from build123d import *

# Parameters (mm, degrees)
F0_R     = 20
F0_R_2   = 2
F0_R_3   = 12.5
F1_DEPTH = 2


with BuildPart() as f1:
    # F0 (on Top) → F1 (new body)
    with BuildSketch(Plane.XY):
        Circle(F0_R)
        with Locations((-11.490485, -11.490485)):
            Circle(F0_R_2, mode=Mode.SUBTRACT)
        with Locations((-6.218606, -15.013042)):
            Circle(F0_R_2, mode=Mode.SUBTRACT)
        with Locations((-15.013042, -6.218606)):
            Circle(F0_R_2, mode=Mode.SUBTRACT)
        with Locations((0, -16.25)):
            Circle(F0_R_2, mode=Mode.SUBTRACT)
        with Locations((6.218606, -15.013042)):
            Circle(F0_R_2, mode=Mode.SUBTRACT)
        with Locations((11.490485, -11.490485)):
            Circle(F0_R_2, mode=Mode.SUBTRACT)
        with Locations((15.013042, -6.218606)):
            Circle(F0_R_2, mode=Mode.SUBTRACT)
        with Locations((-16.25, 0)):
            Circle(F0_R_2, mode=Mode.SUBTRACT)
        with Locations((-15.013042, 6.218606)):
            Circle(F0_R_2, mode=Mode.SUBTRACT)
        with Locations((-11.490485, 11.490485)):
            Circle(F0_R_2, mode=Mode.SUBTRACT)
        with Locations((-6.218606, 15.013042)):
            Circle(F0_R_2, mode=Mode.SUBTRACT)
        Circle(F0_R_3, mode=Mode.SUBTRACT)
        with Locations((16.25, 0)):
            Circle(F0_R_2, mode=Mode.SUBTRACT)
        with Locations((15.013042, 6.218606)):
            Circle(F0_R_2, mode=Mode.SUBTRACT)
        with Locations((0, 16.25)):
            Circle(F0_R_2, mode=Mode.SUBTRACT)
        with Locations((6.218606, 15.013042)):
            Circle(F0_R_2, mode=Mode.SUBTRACT)
        with Locations((11.490485, 11.490485)):
            Circle(F0_R_2, mode=Mode.SUBTRACT)
    extrude(amount=F1_DEPTH)


solid = f1.part
Source: CAD feature listing. Evaluate the final solid. Frame: model axes, mm. Round coordinates to 2 decimals unless told otherwise and drop trailing zeros. Order: outer loops, then holes, each group sorted by start corner. A loop starts at its lowest first (then second) coordinate and runs counter-clockwise, first axis right, second up. Notation, with made-up numbers: (-13, 49.5) - (11, 49.5) arc R37 ccw to (11, 86.5) - close; hole circle Ø8 at (-20, 64). An arc over 180 degrees is marked (long way). Use a Markdown table: item, result. Add a question column.
1. Section query C-C (z = 0.3). Give the number of separate pieces and of enclosed holes in the cut face, then the cut area to 3 significant figures.
2. Mould query, pull axis Y, two halves, no side actions, for faces 1 (the cylindrical face through (-4.336, -19.524, 0.986)), 2 (the flat face through (-9, -9, 2)), 3 (the cylindrical face through (-7.81, 13.8, 0.99)). Classes: +Y half, -Y half, draft (parallel to the pull), parting line (faces both ways), or undercut.
3. Section query D-D (y = 17.5). Return the cut outline in (x, z), then the cut area to 3 significant figures.
4. First-contact query: pin 1 (2 mm diameter, centred on x = -1.5, y = -9.5, fed in from +Z). Flat tip, straight axial feed; report the tip coordinate or a pass-through.
5. Section query A-A (y = 0). Return the cut outline in (x, z).
6. Line query: probe 1 along X at (y, z) = (15.5, 0.15); probe 2 along Y at (x, z) = (14, 0.6); probe 3 along Y at (x, z) = (-7.5, 0.35). Output: solid intervals per line, ascending.
Derived:
| question | item | result |
|---|---|---|
| 1 | separate pieces | 1 |
| 1 | enclosed holes | 17 |
| 1 | area | 565 mm2 |
| 2 | face 1 | parting line |
| 2 | face 2 | draft |
| 2 | face 3 | undercut |
| 3 | outline | (-9.68, 0) - (-1.56, 0) - (-1.56, 2) - (-9.68, 2) - close; (1.56, 0) - (9.68, 0) - (9.68, 2) - (1.56, 2) - close |
| 3 | area | 32.5 mm2 |
| 4 | pin 1 | through |
| 5 | outline | (-20, 0) - (-18.25, 0) - (-18.25, 2) - (-20, 2) - close; (-14.25, 0) - (-12.5, 0) - (-12.5, 2) - (-14.25, 2) - close; (12.5, 0) - (14.25, 0) - (14.25, 2) - (12.5, 2) - close; (18.25, 0) - (20, 0) - (20, 2) - (18.25, 2) - close |
| 6 | probe 1 | -12.64 to -8.16, -4.28 to -1.85, 1.85 to 4.28, 8.16 to 12.64 |
| 6 | probe 2 | -14.28 to -7.94, -4.49 to 4.49, 7.94 to 14.28 |
| 6 | probe 3 | -18.54 to -16.55, -13.48 to -10, 10 to 13.48, 16.55 to 18.54 |
